Input: part model. Units: mm. Frame: model coordinates. A direction names the side the tool comes from. Round coordinates to 2 decimals unless told otherwise and drop trailing zeros. Loops run counter-clockwise (first coordinate to the right, second up) from the corner with the lowest first, then second, coordinate; pieces in that order, holes last. Notation, with made-up numbers: M -39,-28 L 0,-28 A16 cw 0,-24 Z; hole C 60,87 d8. An arc over 180 degrees is marked long. Put each result on its own line as item: value. Start each with the question number.
1) Reachability of faces 1 (the face through (10, 2, -148)), 2 (the face through (0, 48, -74)), 3 (the face through (35, 52, -74)), 4 (the face through (11, 3, -143)) from +Z, -Z, +X, -X, +Y, -Y: full face, straight path, thin tool, end or side. Return the list, or none.
2) Section B-B on x = 27. State how many separate pieces and enclosed holes the cut face has, plus the area to 3 significant figures.
3) Draft query along Y for faces 5 (the face through (22, 0, -76)), 6 (the face through (22.5, 51, -145)), 7 (the face through (35, 80, -74)). Return one class per face: +Y half, -Y half, draft (parallel to the pull), parting line (faces both ways), or undercut.
4) Section C-C on x = 12.5. Output: boundary loops of the cut face in (y, z).
5) Line query: probe 1 along Z at (x, y) = (21.5, 25); probe 2 along X at (y, z) = (42.5, -29). Output: solid intervals per line, ascending.
6) Section A-A on x = 20.5. Output: boundary loops of the cut face in (y, z).
7) Pin query (flat end, axial travel): pin 1 (0.9 mm diameter, centred on y = 63.5, z = -54.5, fed in from +X); pin 2 (11 mm diameter, centred on x = 10, z = -4, fed in from +Y); pin 3 (7 mm diameter, centred on x = 12.5, y = 37, fed in from -Z). Return the tip coordinate at first contact, or that it passes through.
from build123d import *

# Parameters (mm, degrees)
SKETCH1_W           = 45
SKETCH1_H           = 150
BOSS_EXTRUDE1_DEPTH = 97
SKETCH2_W           = 22.5
SKETCH2_H           = 10
CUT_EXTRUDE1_DEPTH  = 94
CUT_EXTRUDE2_DEPTH  = 183.649938407
SKETCH4_W           = 19.5
SKETCH4_H           = 3
CUT_EXTRUDE3_DEPTH  = 185.211834582
LPATTERN1_COUNT     = 19
LPATTERN1_PITCH     = 5


with BuildPart() as part:
    # Sketch1 → Boss-Extrude1 (new body)
    with BuildSketch(Plane(origin=(0, 0, 0), x_dir=(1, 0, 0), z_dir=(0, 1, 0))):
        with Locations((22.5, 75)):
            Rectangle(SKETCH1_W, SKETCH1_H)
    extrude(amount=BOSS_EXTRUDE1_DEPTH)

    # Sketch2 → Cut-Extrude1 (cut)
    with BuildSketch(Plane(origin=(0, 97, 0), x_dir=(1, 0, 0), z_dir=(0, 1, 0))):
        with Locations((11.25, 145)):
            Rectangle(SKETCH2_W, SKETCH2_H)
    cut_extrude1 = extrude(amount=-CUT_EXTRUDE1_DEPTH, mode=Mode.SUBTRACT)

    # Sketch3 → Cut-Extrude2 (cut, through all)
    with BuildSketch(Plane(origin=(0, 3, 0), x_dir=(1, 0, 0), z_dir=(0, 1, 0))):
        with BuildLine():
            Line((10, 150), (10, 146))
            ThreePointArc((10, 146), (12.5, 143.5), (15, 146))
            Line((15, 146), (15, 150))
            Line((15, 150), (10, 150))
        make_face()
    cut_extrude2 = extrude(amount=-CUT_EXTRUDE2_DEPTH, mode=Mode.SUBTRACT)

    # Mirror1: Cut-Extrude1, Cut-Extrude2 across plane
    add(cut_extrude1.mirror(Plane.XY.offset(-75)), mode=Mode.SUBTRACT)
    add(cut_extrude2.mirror(Plane.XY.offset(-75)), mode=Mode.SUBTRACT)

    # Sketch4 → Cut-Extrude3 (cut, through all)
    with BuildSketch(Plane.XY):
        with Locations((35.25, 93.5)):
            Rectangle(SKETCH4_W, SKETCH4_H)
    cut_extrude3 = extrude(amount=-CUT_EXTRUDE3_DEPTH, mode=Mode.SUBTRACT)

    # LPattern1: Cut-Extrude3 ×19
    with Locations(*[(0, -i * LPATTERN1_PITCH, 0) for i in range(1, LPATTERN1_COUNT)]):
        add(cut_extrude3, mode=Mode.SUBTRACT)


solid = part.part
Geometry results:
1. face 1: -Z, +Y, -Y
1. face 2: +Z, -Z, -X, +Y, -Y
1. face 3: +Z, -Z, +X
1. face 4: -Z, -X, +Y
2. separate pieces: 20
2. enclosed holes: 0
2. area: 6,000 mm²
3. face 5: -Y half
3. face 6: draft
3. face 7: undercut
4. outline: M 0,-143.5 L 3,-143.5 L 3,-140 L 97,-140 L 97,-10 L 3,-10 L 3,-6.5 L 0,-6.5 Z
5. probe 1: z = -140 to -10
5. probe 2: x = 0 to 25.5
6. outline: M 0,-150 L 3,-150 L 3,-140 L 97,-140 L 97,-10 L 3,-10 L 3,0 L 0,0 Z
7. pin 1: stops at x = 25.5
7. pin 2: stops at y = 3
7. pin 3: stops at z = -140
